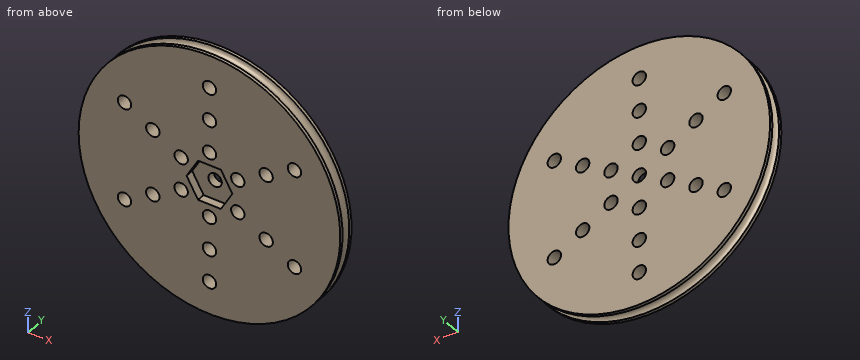
```python
from build123d import *

# Parameters (mm, degrees)
SKETCH001_R        = 2.05
POCKET_DEPTH       = 231.496034
POLARPATTERN_COUNT = 6
POCKET001_DEPTH    = 2.5


with BuildPart() as part:
    # Sketch → Revolution (revolve)
    with BuildSketch(Plane.XY):
        with BuildLine():
            Line((-2.05, 2.5), (-2.05, -2.5))
            Line((-2.05, -2.5), (-40, -2.5))
            Line((-40, -2.5), (-40, -1.5))
            ThreePointArc((-40, -1.5), (-38.5, 0), (-40, 1.5))
            Line((-40, 1.5), (-40, 2.5))
            Line((-40, 2.5), (-2.05, 2.5))
        make_face()
    revolve(axis=Axis((0, 0, 0), (0, 1, 0)))

    # Sketch001 → Pocket (cut, through all)
    with BuildSketch(Plane.XZ.offset(2.5)):
        with Locations((0, 10)):
            Circle(SKETCH001_R)
        with Locations((0, 20)):
            Circle(SKETCH001_R)
        with Locations((0, 30)):
            Circle(SKETCH001_R)
    pocket = extrude(amount=-POCKET_DEPTH, mode=Mode.SUBTRACT)

    # PolarPattern: Pocket ×6 about axis
    polarpattern_axis = Axis((0, -2.5, 0), (0, -1, 0))
    for i in range(1, POLARPATTERN_COUNT):
        add(pocket.rotate(polarpattern_axis, i * 360 / POLARPATTERN_COUNT), mode=Mode.SUBTRACT)

    # Sketch002 → Pocket001 (cut)
    with BuildSketch(Plane.XZ.offset(2.5)):
        Polygon((3.5, -6.062178), (7, 0), (3.5, 6.062178), (-3.5, 6.062178), (-7, 0), (-3.5, -6.062178), align=None)
    extrude(amount=-POCKET001_DEPTH, mode=Mode.SUBTRACT)


solid = part.part
```
Verification items for the finished model (mm, model axes). Coordinates: 2 decimals unless noted, no trailing zeros. Put each result on its own line as item: value.
1. Thickness scan on line 1 (Z direction, x = 17, y = -1.95); line 2 (Z direction, x = -8, y = -2.2); line 3 (X direction, y = 1.6, z = -13.5). Record the ranges inside material, lowest first.
Result set:
line 1: z = -36.21 to -12.02, -7.98 to 7.98, 12.02 to 36.21
line 2: z = -39.19 to -6.94, -3.06 to 3.06, 6.94 to 39.19
line 3: x = -37.65 to -27.38, -24.58 to 24.58, 27.38 to 37.65
2. Gauge pin test, flat ends, axial feed: P1, Ø0.8, axis at x = 1, y = -1.5, coming from the +Z side; P2, Ø1, axis at x = 4, y = -0.5, coming from the -Z side; P3, Ø3, axis at y = 0.5, z = -16, coming from the -X side. Record the tip position at first contact, or that the pin passes through.
Result set:
P1: stops at z = 40
P2: stops at z = -38.68
P3: stops at x = -37.13
3. Section check A-A, the plane z = -5. Give the number of separate pieces and of enclosed holes in the cut face, then the cut area to 3 significant figures.
Result set:
separate pieces: 3
enclosed holes: 0
area: 328 mm^2
